Verification items for the finished model (mm, model axes). A direction names the side the tool comes from. Round coordinates to 2 decimals unless told otherwise and drop trailing zeros. Order: outer loops, then holes, each group sorted by start corner. A loop starts at its lowest first (then second) coordinate and runs counter-clockwise, first axis right, second up. Notation, with made-up numbers: M -36.75,35.25 L 3.25,35.25 A13 ccw 3.25,56.25 Z; hole C -5,84.5 d6. An arc over 180 degrees is marked long. One line per item, written item: value. Start each with the question number.
from build123d import *
from build123d.topology import SkipClean

# Parameters (mm, degrees)
SKETCH1_W           = 55
SKETCH1_H           = 10
SKETCH1_R           = 1.5
BOSS_EXTRUDE1_DEPTH = 15
BOSS_EXTRUDE2_START = 3
SKETCH2_W           = 25
SKETCH2_H           = 10
SKETCH2_R           = 1.5
SKETCH2_W_2         = 15
BOSS_EXTRUDE2_DEPTH = 3


with BuildPart() as part:
    # Sketch1 → Boss-Extrude1 (new body)
    with BuildSketch(Plane.XY):
        with Locations((-27.5, 5)):
            Rectangle(SKETCH1_W, SKETCH1_H)
        with Locations((-2.5, 5)):
            Circle(SKETCH1_R, mode=Mode.SUBTRACT)
        with Locations((-12.5, 5)):
            Circle(SKETCH1_R, mode=Mode.SUBTRACT)
        with Locations((-42.5, 5)):
            Circle(SKETCH1_R, mode=Mode.SUBTRACT)
        with Locations((-52.5, 5)):
            Circle(SKETCH1_R, mode=Mode.SUBTRACT)
    extrude(amount=BOSS_EXTRUDE1_DEPTH)

    # Sketch2 → Boss-Extrude2 (add)
    # profile 1 of 5: a face of its own
    with SkipClean():  # the faces are left unmerged after this step: merging them gives an invalid solid
        with BuildSketch(Plane(origin=(0, 0, 0), x_dir=(-1, 0, 0), z_dir=(0, 0, -1)).offset(BOSS_EXTRUDE2_START)):
            with Locations((27.5, 5)):
                Rectangle(SKETCH2_W, SKETCH2_H)
        # profile 2 of 5: a face of its own
        with BuildSketch(Plane(origin=(0, 0, 0), x_dir=(-1, 0, 0), z_dir=(0, 0, -1)).offset(BOSS_EXTRUDE2_START)):
            with BuildLine():
                Line((0, 55), (0, 10))
                Line((0, 10), (15, 10))
                Line((15, 10), (15, 19.850540474))
                ThreePointArc((15, 19.850540474), (14, 22.300030217), (15, 24.74951996))
                Line((15, 24.74951996), (15, 55))
                Line((15, 55), (0, 55))
            make_face()
            with Locations((2.5, 50)):
                Circle(SKETCH2_R, mode=Mode.SUBTRACT)
            with Locations((12.5, 50)):
                Circle(SKETCH2_R, mode=Mode.SUBTRACT)
        # profile 3 of 5: a face of its own
        with BuildSketch(Plane(origin=(0, 0, 0), x_dir=(-1, 0, 0), z_dir=(0, 0, -1)).offset(BOSS_EXTRUDE2_START)):
            with Locations((7.5, 5)):
                Rectangle(SKETCH2_W_2, SKETCH2_H)
            with Locations((2.5, 5)):
                Circle(SKETCH2_R, mode=Mode.SUBTRACT)
            with Locations((12.5, 5)):
                Circle(SKETCH2_R, mode=Mode.SUBTRACT)
        # profile 4 of 5: a face of its own
        with BuildSketch(Plane(origin=(0, 0, 0), x_dir=(-1, 0, 0), z_dir=(0, 0, -1)).offset(BOSS_EXTRUDE2_START)):
            with Locations((47.5, 5)):
                Rectangle(SKETCH2_W_2, SKETCH2_H)
            with Locations((42.5, 5)):
                Circle(SKETCH2_R, mode=Mode.SUBTRACT)
            with Locations((52.5, 5)):
                Circle(SKETCH2_R, mode=Mode.SUBTRACT)
        # profile 5 of 5: a face of its own
        with BuildSketch(Plane(origin=(0, 0, 0), x_dir=(-1, 0, 0), z_dir=(0, 0, -1)).offset(BOSS_EXTRUDE2_START)):
            with BuildLine():
                Line((40, 19.850540474), (40, 10))
                Line((40, 10), (55, 10))
                Line((55, 10), (55, 55))
                Line((55, 55), (40, 55))
                Line((40, 55), (40, 24.74951996))
                ThreePointArc((40, 24.74951996), (40.740370349, 23.622905872), (41, 22.300030217))
                ThreePointArc((41, 22.300030217), (40.740370349, 20.977154561), (40, 19.850540474))
            make_face()
            with Locations((42.5, 50)):
                Circle(SKETCH2_R, mode=Mode.SUBTRACT)
            with Locations((52.5, 50)):
                Circle(SKETCH2_R, mode=Mode.SUBTRACT)
        extrude(amount=-BOSS_EXTRUDE2_DEPTH)


solid = part.part
1. Scan lines: line 1 along X through (y, z) = (5, 9.5); line 2 along X through (y, z) = (25.5, -1.5); line 3 along Z through (x, y) = (-3.5, 28). Record each from-to range of solid material in increasing order.
2. Draft check along X on faces 1 (the face through (-41.3, 49.1, -1.5)), 2 (the face through (-55, 15, -2)), 3 (the face through (-48, 55, -2)). Enter one of: released by +X, released by -X, zero draft, split by the parting line, or undercut.
3. Section check C-C (z = 3). Record the cut outline in (x, y).
4. Section check A-A (y = 50). Record the cut outline in (x, z).
5. Section check D-D (y = 31). Record the cut outline in (x, z), and give its area (3 significant figures).
6. Depth check by flat-ended pin: pin 1 (3.5 mm diameter, centred on x = -12.5, y = 5, fed in from +Z); pin 2 (12 mm diameter, centred on x = -10, y = 30.5, fed in from +Z); pin 3 (2 mm diameter, centred on x = -17, y = 22.5, fed in from -Z); pin 4 (1.5 mm diameter, centred on x = -29.5, z = 3, fed in from +Y). Enter the tip coordinate at first touch or a pass-through.
7. Tool access check on faces 4 (the face through (-28, 5, 15)), 5 (the face through (-47, 33, 0)), 6 (the face through (0, 15, -2)), 7 (the face through (-15, 40, -2)), 8 (the face through (-14, 22.3, -1.5)). Record the directions out of +Z, -Z, +X, -X, +Y, -Y that give a thin tool (end or side, any length) a straight path to the whole face; none if there is none.
Geometry check:
1. line 1: x = -55 to -54, -51 to -44, -41 to -14, -11 to -4, -1 to 0
1. line 2: x = -55 to -40, -15 to 0
1. line 3: z = -3 to 0
2. face 1: undercut
2. face 2: released by -X
2. face 3: zero draft
3. outline: M -55,0 L 0,0 L 0,10 L -55,10 Z; hole C -52.5,5 d3; hole C -42.5,5 d3; hole C -12.5,5 d3; hole C -2.5,5 d3
4. outline: M -55,-3 L -54,-3 L -54,0 L -55,0 Z; M -51,-3 L -44,-3 L -44,0 L -51,0 Z; M -41,-3 L -40,-3 L -40,0 L -41,0 Z; M -15,-3 L -14,-3 L -14,0 L -15,0 Z; M -11,-3 L -4,-3 L -4,0 L -11,0 Z; M -1,-3 L 0,-3 L 0,0 L -1,0 Z
5. outline: M -55,-3 L -40,-3 L -40,0 L -55,0 Z; M -15,-3 L 0,-3 L 0,0 L -15,0 Z
5. area: 90.0 mm²
6. pin 1: stops at z = 15
6. pin 2: stops at z = 0
6. pin 3: passes through
6. pin 4: stops at y = 10
7. face 4: +Z, +X, -X, +Y, -Y
7. face 5: +Z, +X, -X, +Y
7. face 6: +Z, -Z, +X, +Y, -Y
7. face 7: +Z, -Z, +Y
7. face 8: +Z, -Z
